```python
from build123d import *

# Parameters (mm, degrees)
F1_DEPTH  = 15
F3_DEPTH  = 50
F4_DEPTH  = 5
F6_DEPTH  = 34.1
F8_DEPTH  = 5
F10_DEPTH = 37.3
F11_DEPTH = 10
F12_DEPTH = 10
F13_DEPTH = 25
F14_DEPTH = 25


with BuildPart() as f1:
    # F0 (on Top) → F1 (new body)
    with BuildSketch(Plane.XY):
        Polygon((50, 0), (0, 0), (0, -10), (60, -10), (60, 50), (50, 50), align=None)
    extrude(amount=F1_DEPTH)

    # F2 (on face) → F3 (join)
    with BuildSketch(Plane(origin=(50, 0, 0), x_dir=(0, -1, 0), z_dir=(-1, 0, 0))):
        Polygon((-50, 10), (-50, 5), (0, 5), (0, 10), (-10, 10), (-14.4219835103, 10), (-35, 10), (-40, 10), align=None)
    extrude(amount=F3_DEPTH)

    # F2 (on face) → F4 (join)
    with BuildSketch(Plane(origin=(50, 0, 0), x_dir=(0, -1, 0), z_dir=(-1, 0, 0))):
        Polygon((-40, 15), (-40, 10), (-35, 10), (-35, 15), (-37.5, 15), align=None)
        Polygon((-14.4219835103, 10), (-10, 10), (-10, 15), (-12.5, 15), (-14.4219835103, 15), align=None)
    extrude(amount=F4_DEPTH)

    # F5 (on face) → F6 (cut)
    with BuildSketch(Plane(origin=(0, 40, 0), x_dir=(-1, 0, 0), z_dir=(0, 1, 0))):
        Polygon((-45, 15), (-50, 15), (-45, 10), align=None)
    extrude(amount=-F6_DEPTH, mode=Mode.SUBTRACT)

    # F7 (on face) → F8 (join)
    with BuildSketch(Plane(origin=(0, 0, 0), x_dir=(-1, 0, 0), z_dir=(0, 1, 0))):
        Polygon((-40, 15), (-40, 10), (-35, 10), (-35, 15), (-37.5, 15), align=None)
        Polygon((-15, 15), (-15, 10), (-10, 10), (-10, 15), (-12.5, 15), align=None)
    extrude(amount=F8_DEPTH)

    # F9 (on face) → F10 (cut)
    with BuildSketch(Plane(origin=(10, 0, 0), x_dir=(0, -1, 0), z_dir=(-1, 0, 0))):
        Polygon((-5, 15), (-5, 10), (0, 15), align=None)
    extrude(amount=-F10_DEPTH, mode=Mode.SUBTRACT)

    # F2 (on face) → F11 (join)
    with BuildSketch(Plane(origin=(50, 0, 0), x_dir=(0, -1, 0), z_dir=(-1, 0, 0))):
        with BuildLine():
            Line((-35, 20), (-35, 15))
            Line((-35, 15), (-26.5, 15))
            ThreePointArc((-26.5, 15), (-25, 16.5), (-23.5, 15))
            Line((-23.5, 15), (-14.4219835103, 15))
            Line((-14.4219835103, 15), (-19.4219835103, 20))
            Line((-19.4219835103, 20), (-35, 20))
        make_face()
    extrude(amount=-F11_DEPTH)

    # F7 (on face) → F12 (join)
    with BuildSketch(Plane(origin=(0, 0, 0), x_dir=(-1, 0, 0), z_dir=(0, 1, 0))):
        with BuildLine():
            Line((-30, 20), (-35, 15))
            Line((-35, 15), (-26.5, 15))
            ThreePointArc((-26.5, 15), (-25, 16.5), (-23.5, 15))
            Line((-23.5, 15), (-15, 15))
            Line((-15, 15), (-15, 20))
            Line((-15, 20), (-30, 20))
        make_face()
    extrude(amount=-F12_DEPTH)

    # F2 (on face) → F13 (cut)
    with BuildSketch(Plane(origin=(50, 0, 0), x_dir=(0, -1, 0), z_dir=(-1, 0, 0))):
        with BuildLine():
            Line((-23.5, 15), (-26.5, 15))
            ThreePointArc((-26.5, 15), (-25, 13.5), (-23.5, 15))
        make_face()
        with BuildLine():
            ThreePointArc((-23.5, 15), (-25, 16.5), (-26.5, 15))
            Line((-26.5, 15), (-23.5, 15))
        make_face()
    extrude(amount=-F13_DEPTH, mode=Mode.SUBTRACT)

    # F7 (on face) → F14 (cut)
    with BuildSketch(Plane(origin=(0, 0, 0), x_dir=(-1, 0, 0), z_dir=(0, 1, 0))):
        with BuildLine():
            ThreePointArc((-23.5, 15), (-25, 16.5), (-26.5, 15))
            Line((-26.5, 15), (-23.5, 15))
        make_face()
        with BuildLine():
            Line((-23.5, 15), (-26.5, 15))
            ThreePointArc((-26.5, 15), (-25, 13.5), (-23.5, 15))
        make_face()
    extrude(amount=-F14_DEPTH, mode=Mode.SUBTRACT)


solid = f1.part
```
The model under review builds one solid part; all positions refer to its coordinate system, in mm. A direction names the side the tool comes from. Give positions to 0.01 mm unless a question says otherwise; leave off trailing zeros. Write each loop counter-clockwise with the first axis right and the second up, starting at its lowest first coordinate (ties: lowest second). Pieces come first, ordered by that corner, then holes. Notation, with made-up numbers: (34, 83.25) - (91, 83.25) arc R12 ccw to (91, 98.25) - close; hole circle Ø10 at (-12, 72). An arc over 180 degrees is marked (long way). Answer in a Markdown table with one row per item. Add a question column.
1. We need section D-D on z = 3.25. Write out the cut boundary in (x, y), then the cut area to 3 significant figures.
2. Tool access review of faces 4 (the flat face through (10, 2, 12)), 5 (the flat face through (48, 35, 12)), 6 (the flat face through (45, 0, 12)), 7 (the flat face through (25, 25, 5)): name each direction out of +Z, -Z, +X, -X, +Y, -Y from which nothing blocks a thin tool from reaching the whole face with its end or side.
3. Wall thickness on line 1 along Z through (x, y) = (25, -2.25); line 2 along Y through (x, z) = (36.5, 3.75); line 3 along X through (y, z) = (29.5, 12.25): over which ranges is each line inside the solid? List them lowest first. Write a range as [from, to].
4. Insertion check: P1, Ø1.5, axis at x = 46.5, z = 13.5, coming from the +Y side; P2, Ø5.5, axis at y = 46, z = 12, coming from the -X side; P3, Ø2.5, axis at y = 20.5, z = 3.5, coming from the -X side; P4, Ø10, axis at x = 21.5, y = 39, coming from the +Z side. Each pin has a flat end and moves straight along its axis. Give the tip position at first contact, or say it passes through.
5. We need section B-B on x = 25. Write out the cut boundary in (y, z).
6. Draft analysis for pull direction X (two halves, no side actions). For faces 1 (the flat face through (0, 14, 7)), 2 (the flat face through (37, 50, 7)), 3 (the flat face through (15, 1, 11)), state which applies: +X half, -X half, draft (parallel to the pull), parting line (faces both ways), or undercut.
7. We need section A-A on y = 25. Write out the cut boundary in (x, z), then the cut area to 3 significant figures.
8. We need section C-C on x = 48. Write out the cut boundary in (y, z).
Ans:
| question | item | result |
|---|---|---|
| 1 | outline | (0, -10) - (60, -10) - (60, 50) - (50, 50) - (50, 0) - (0, 0) - close |
| 1 | area | 1,100 mm^2 |
| 2 | face 4 | +Z, -X, +Y |
| 2 | face 5 | +Z, -X |
| 2 | face 6 | +Z |
| 2 | face 7 | -Z, -X, +Y |
| 3 | line 1 | z = [0, 13.5], [16.5, 20] |
| 3 | line 2 | y = [-10, 0] |
| 3 | line 3 | x = [50, 60] |
| 4 | P1 | stops at y = 0 |
| 4 | P2 | stops at x = 0 |
| 4 | P3 | stops at x = 50 |
| 4 | P4 | stops at z = 10 |
| 5 | outline | (-10, 0) - (0, 0) - (0, 5) - (50, 5) - (50, 10) - (0, 10) - (0, 13.5) - (-10, 13.5) - close; (-10, 16.5) - (0, 16.5) - (0, 20) - (-10, 20) - close |
| 6 | face 1 | -X half |
| 6 | face 2 | draft |
| 6 | face 3 | undercut |
| 7 | outline | (0, 5) - (50, 5) - (50, 0) - (60, 0) - (60, 13.5) - (50, 13.5) - (50, 10) - (0, 10) - close; (50, 16.5) - (60, 16.5) - (60, 20) - (50, 20) - close |
| 7 | area | 420 mm^2 |
| 8 | outline | (-10, 0) - (0, 0) - (0, 5) - (50, 5) - (50, 10) - (40, 10) - (40, 13) - (35, 13) - (35, 10) - (14.42, 10) - (14.42, 13) - (10, 13) - (10, 10) - (0, 10) - (0, 15) - (-10, 15) - close |
